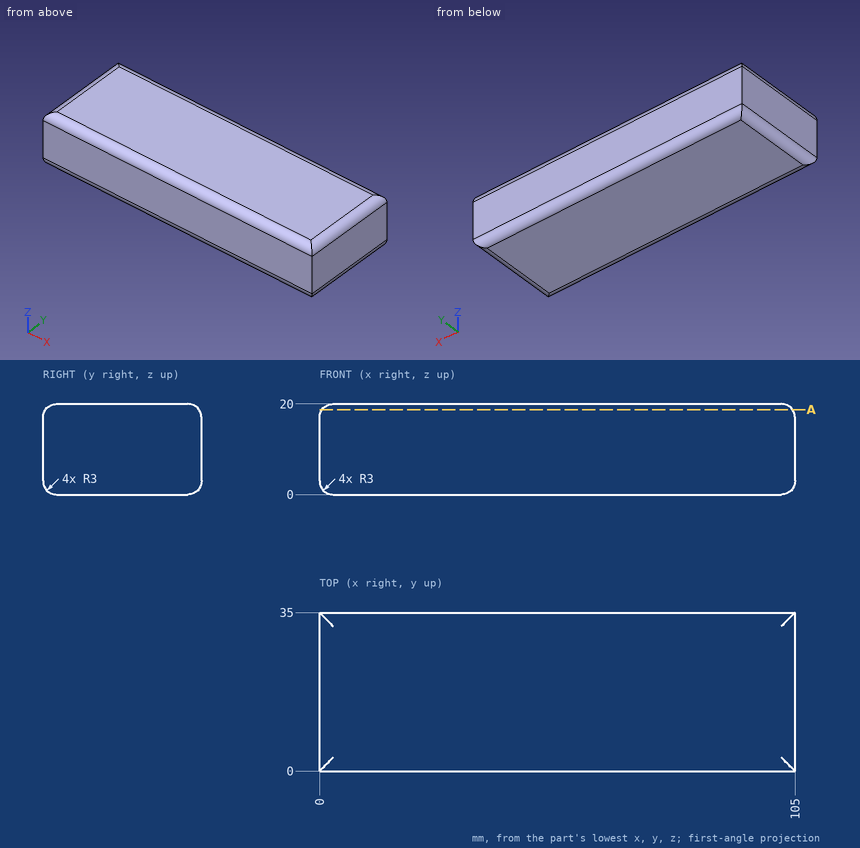
Can you work these out from the drawing? Everything is in mm from the part's minimum corner. Coordinates: 2 decimals unless noted, no trailing zeros. Loops run counter-clockwise (first coordinate to the right, second up) from the corner with the lowest first, then second, coordinate; pieces in that order, holes last.
1. I need wall thicknesses on L1, parallel to Y at x = 22, z = 2.75; L2, parallel to Y at x = 93, z = 2; L3, parallel to X at y = 21.5, z = 17.75. Which ranges of each line are inside material? Lowest first, please.
2. Imagine slicing it at A-A, the plane z = 18.75. Please give me the cut outline in (x, y), and give its area (3 significant figures).
3. For P1, Ø1.5, axis at y = 31, z = 2, coming from the -X side, with a flat end and sliding along its axis, tell me the tip position at first contact or that it passes through.
Taken from the geometry:
1. L1: y = 0.01 to 34.99
1. L2: y = 0.17 to 34.83
1. L3: x = 0.1 to 104.9
2. outline: (0.56, 0.56) - (104.44, 0.56) - (104.44, 34.44) - (0.56, 34.44) - close
2. area: 3,520 mm2
3. P1: stops at x = 0.01
